```python
from build123d import *

# Parameters (mm, degrees)
SKETCH2_W           = 5
SKETCH2_H           = 5
FILLET1_R           = 2.5
BOSS_EXTRUDE1_DEPTH = 5


with BuildPart() as part:
    # Sweep1: sweep along a path in Sketch1
    with BuildLine(Plane(origin=(0, 0, 0), x_dir=(1, 0, 0), z_dir=(0, 1, 0))) as sweep1_path:
        Line((0, -14.5), (0, 14.5))
        Line((0, 14.5), (-25, 14.5))
        ThreePointArc((-25, 14.5), (-33.507810594, 15.992189406), (-41, 20.290627288))
        Line((-41, 20.290627288), (-44.841874542, 23.490627288))
    # Sketch2 → Sweep1 (sweep)
    with BuildSketch(Plane.XY.offset(14.5)):
        Rectangle(SKETCH2_W, SKETCH2_H)
    sweep(path=sweep1_path.line, transition=Transition.RIGHT)

    # Fillet1
    fillet1_edges = [part.edges().sort_by_distance(p)[0] for p in [
        (-41.320937271, -2.5, -23.811564559),
        (-32.657029534, -2.5, -18.342970466),
        (-41.320937271, 2.5, -23.811564559),
        (-32.657029534, 2.5, -18.342970466),
        (-11.25, -2.5, -17),
        (-11.25, 2.5, -17),
    ]]
    fillet(fillet1_edges, radius=FILLET1_R - 0.0001)  # a hair under: the kernel refuses the full size

    # Sketch3 → Boss-Extrude1 (add)
    with BuildSketch(Plane(origin=(0, 2.5, 0), x_dir=(1, 0, 0), z_dir=(0, 1, 0))):
        Polygon((-17.029574207, 12), (-2.5, -5.112609621), (-2.5, -1.25), (-13.75, 12), align=None)
    extrude(amount=-BOSS_EXTRUDE1_DEPTH)


solid = part.part
```
The model under review builds one solid part; all positions refer to its coordinate system, in mm. A direction names the side the tool comes from. Round coordinates to 2 decimals unless told otherwise and drop trailing zeros. Loops run counter-clockwise (first coordinate to the right, second up) from the corner with the lowest first, then second, coordinate; pieces in that order, holes last. Notation, with made-up numbers: (-7, 43) -> (11, 43) arc R22 cw to (11, 71) -> close; hole circle Ø3 at (44.5, 14). An arc over 180 degrees is marked (long way). Answer in a Markdown table with one row per item.
1) Tool access review of faces 5 (the flat face through (-21, 0, -12)), 6 (the cylindrical face through (-11, -2, -16)), 7 (the flat face through (-8.046, 0.035, -5.282)): name each direction out of +Z, -Z, +X, -X, +Y, -Y from which nothing blocks a thin tool from reaching the whole face with its end or side.
Taken from the geometry:
| item | result |
|---|---|
| face 5 | +Z, -X, +Y, -Y |
| face 6 | -Z, +X, -Y |
| face 7 | +Y, -Y |
2) Consider section A-A, the plane z = -2. Write out the cut boundary in (x, y).
Taken from the geometry:
| item | result |
|---|---|
| outline | (-8.54, -2.5) -> (-5.26, -2.5) -> (-5.26, 2.5) -> (-8.54, 2.5) -> close; (-2.5, -2.5) -> (2.5, -2.5) -> (2.5, 2.5) -> (-2.5, 2.5) -> close |
3) For pin 1 Ø1 at (x, y) = (-15.5, -1.5) entering from -Z; pin 2 Ø12 at (x, z) = (-34, -2) entering from +Y; pin 3 Ø2 at (y, z) = (-1, -8.5) entering from -X; pin 4 Ø1 at (x, z) = (-31, -17.5) entering from -Y, all flat-tipped, find the tip position at first contact; note any pin that passes through.
Taken from the geometry:
| item | result |
|---|---|
| pin 1 | stops at z = -16.79 |
| pin 2 | passes through |
| pin 3 | stops at x = -14.91 |
| pin 4 | stops at y = -1.84 |
4) Draft analysis for pull direction Z (two halves, no side actions). For faces 1 (the flat face through (2.5, 0, -1)), 2 (the flat face through (0, 0, 14.5)), 3 (the flat face through (-8, 0, -12)), 4 (the cylindrical face through (-41.829, -1.787, -23.256)), state which applies: pulls with the +Z half, pulls with the -Z half, needs draft (parallel to the pull), parting line crosses it, or undercut.
Taken from the geometry:
| item | result |
|---|---|
| face 1 | needs draft |
| face 2 | pulls with the +Z half |
| face 3 | undercut |
| face 4 | pulls with the -Z half |
5) Wall thickness on line 1 along X through (y, z) = (0.75, -6); line 2 along X through (y, z) = (-2, -1.5); line 3 along X through (y, z) = (1.75, 13): over which ranges is each line inside the solid? List them lowest first.
Taken from the geometry:
| item | result |
|---|---|
| line 1 | x = -11.94 to -8.66, -2.5 to 2.5 |
| line 2 | x = -8.11 to -4.83, -2.5 to 2.5 |
| line 3 | x = -2.5 to 2.5 |
6) Consider section C-C, the plane y = -1.2. Write out the cut boundary in (x, z), plus the area to 3 significant figures.
Taken from the geometry:
| item | result |
|---|---|
| outline | (-46.44, -21.57) -> (-43.44, -25.18) -> (-39.6, -21.98) arc R22.81 cw to (-25, -16.69) -> (2.5, -16.69) -> (2.5, 14.5) -> (-2.5, 14.5) -> (-2.5, 5.11) -> (-17.03, -12) -> (-25, -12) arc R27.5 ccw to (-42.6, -18.37) -> close; hole (-13.75, -12) -> (-2.5, -12) -> (-2.5, 1.25) -> close |
| area | 417 mm² |
